Source: CAD feature listing. Evaluate the final solid. Frame: model axes, mm. Give positions to 0.01 mm unless a question says otherwise; leave off trailing zeros. Loops run counter-clockwise (first coordinate to the right, second up) from the corner with the lowest first, then second, coordinate; pieces in that order, holes last. Notation, with made-up numbers: M 37,32.5 L 66,32.5 A23 ccw 66,51.5 Z; hole C 52.5,-38 d4. An arc over 180 degrees is marked long. Put each result on its own line as item: value. Start each with the question number.
```python
from build123d import *

# Parameters (mm, degrees)
SKETCH_1_R          = 2
EXTRUDE_1_DEPTH     = 5
SKETCH_5_R          = 1.5
SKETCH_5_W          = 16.1
SKETCH_5_H          = 16.1
CUT_EXTRUDE_1_DEPTH = 4
EXTRUDE_2_DEPTH     = 5
FILLET_1_R          = 2
SKETCH_9_R          = 1.5
CUT_EXTRUDE_2_DEPTH = 10


with BuildPart() as part:
    # 草图1 → 凸台-拉伸1 (new body)
    with BuildSketch(Plane.XY):
        with BuildLine():
            Line((62.7093167, -58.345136948), (62.7093167, 57.654863052))
            ThreePointArc((62.7093167, 57.654863052), (62.123530262, 59.069076614), (60.7093167, 59.654863052))
            Line((60.7093167, 59.654863052), (-54.2906833, 59.654863052))
            ThreePointArc((-54.2906833, 59.654863052), (-55.704896862, 59.069076614), (-56.2906833, 57.654863052))
            Line((-56.2906833, 57.654863052), (-56.2906833, -58.345136948))
            ThreePointArc((-56.2906833, -58.345136948), (-55.704896862, -59.759350511), (-54.2906833, -60.345136948))
            Line((-54.2906833, -60.345136948), (60.7093167, -60.345136948))
            ThreePointArc((60.7093167, -60.345136948), (62.123530262, -59.759350511), (62.7093167, -58.345136948))
        make_face()
        with Locations((-52.2906833, -56.345136948)):
            Circle(SKETCH_1_R, mode=Mode.SUBTRACT)
        with Locations((58.7093167, -56.345136948)):
            Circle(SKETCH_1_R, mode=Mode.SUBTRACT)
        with Locations((58.7093167, 55.654863052)):
            Circle(SKETCH_1_R, mode=Mode.SUBTRACT)
        with Locations((-52.2906833, 55.654863052)):
            Circle(SKETCH_1_R, mode=Mode.SUBTRACT)
    extrude(amount=EXTRUDE_1_DEPTH)

    # 草图5 → 切除-拉伸1 (cut, through all)
    with BuildSketch(Plane.XY.offset(3)):
        with Locations((-48.275635297, 18.301860934)):
            Circle(SKETCH_5_R)
        with Locations((50.252991339, 18.301860934)):
            Circle(SKETCH_5_R)
        with Locations((-48.275635297, -6.698139066)):
            Circle(SKETCH_5_R)
        with Locations((50.252991339, -6.698139066)):
            Circle(SKETCH_5_R)
        with Locations((-48.275635297, -31.698139066)):
            Circle(SKETCH_5_R)
        with Locations((50.252991339, -31.698139066)):
            Circle(SKETCH_5_R)
        with Locations((25.214825615, -7.576393001)):
            Rectangle(SKETCH_5_W, SKETCH_5_H)
        with Locations((25.214825615, 14.423606999)):
            Rectangle(SKETCH_5_W, SKETCH_5_H)
        with Locations((3.214825615, -7.576393001)):
            Rectangle(SKETCH_5_W, SKETCH_5_H)
        with Locations((-18.785174385, 14.423606999)):
            Rectangle(SKETCH_5_W, SKETCH_5_H)
        with Locations((-18.785174385, -7.576393001)):
            Rectangle(SKETCH_5_W, SKETCH_5_H)
        with Locations((-18.785174385, -29.576393001)):
            Rectangle(SKETCH_5_W, SKETCH_5_H)
        with Locations((3.214825615, 14.423606999)):
            Rectangle(SKETCH_5_W, SKETCH_5_H)
        with Locations((3.214825615, -29.576393001)):
            Rectangle(SKETCH_5_W, SKETCH_5_H)
        with Locations((25.214825615, -29.576393001)):
            Rectangle(SKETCH_5_W, SKETCH_5_H)
        with Locations((25.214825615, -50.576393001)):
            Rectangle(SKETCH_5_W, SKETCH_5_H)
        with Locations((3.214825615, -50.576393001)):
            Rectangle(SKETCH_5_W, SKETCH_5_H)
        with Locations((-18.785174385, -50.576393001)):
            Rectangle(SKETCH_5_W, SKETCH_5_H)
    extrude(amount=-CUT_EXTRUDE_1_DEPTH, mode=Mode.SUBTRACT)

    # 草图8 → 凸台-拉伸2 (add)
    with BuildSketch(Plane.XY.offset(5)):
        Polygon((-56.2906833, -58.345136948), (-26.835174385, -58.345136948), (-26.835174385, -60.345136948), (33.264825615, -60.345136948), (33.264825615, -58.345136948), (62.7093167, -58.345136948), (62.7093167, -68.345136948), (33.264825615, -68.345136948), (-26.835174385, -68.345136948), (-56.2906833, -68.345136948), align=None)
    extrude(amount=-EXTRUDE_2_DEPTH)

    # 圆角1
    fillet_1_edges = [part.edges().sort_by_distance(p)[0] for p in [
        (-56.2906833, -68.345136948, 2.5),
        (62.7093167, -68.345136948, 2.5),
    ]]
    fillet(fillet_1_edges, radius=FILLET_1_R)

    # 草图9 → 切除-拉伸2 (cut)
    with BuildSketch(Plane(origin=(0, 0, 0), x_dir=(-1, 0, 0), z_dir=(0, 0, -1))):
        with Locations((-50.252991339, -6.698139066)):
            Circle(SKETCH_9_R)
        with Locations((-50.252991339, -31.698139066)):
            Circle(SKETCH_9_R)
        with Locations((48.275635297, -31.698139066)):
            Circle(SKETCH_9_R)
        with Locations((48.275635297, -6.698139066)):
            Circle(SKETCH_9_R)
        with Locations((48.275635297, 18.301860934)):
            Circle(SKETCH_9_R)
        with Locations((-50.252991339, 18.301860934)):
            Circle(SKETCH_9_R)
    extrude(amount=-CUT_EXTRUDE_2_DEPTH, mode=Mode.SUBTRACT)


solid = part.part
```
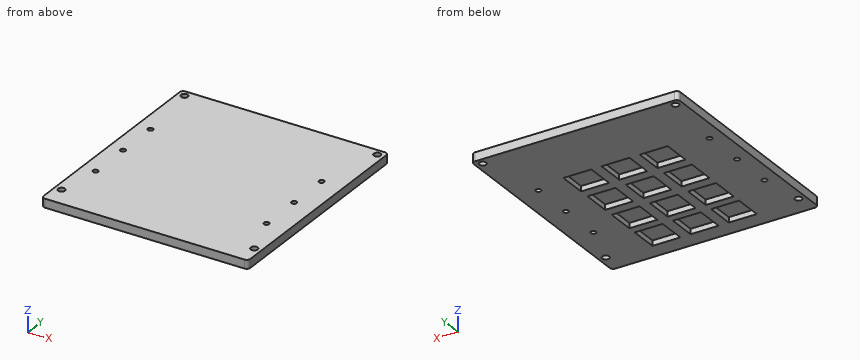
1. Section B-B, the plane y = -48. Output: boundary loops of the cut face in (x, z).
2. Contact query for flat-ended pins moving along their axis: pin 1 (1.8 mm diameter, centred on x = -48.28, y = -31.7, fed in from +Z); pin 2 (8 mm diameter, centred on x = 2, y = -8, fed in from -Z). Output: stop coordinate, or through.
3. Ray query, line 1 (Y direction, x = 4, z = 1.35); line 2 (X direction, y = -2.5, z = 2.55); line 3 (X direction, y = 18, z = 0.75). Return the intervals inside material, ascending.
4. Section C-C, the plane z = 1.45. State how many separate pieces and enclosed holes the cut face has, plus the area to 3 significant figures.
5. Section A-A, the plane x = 25.5. Output: boundary loops of the cut face in (y, z).
Results found:
1. outline: M -56.29,0 L -26.84,0 L -26.84,3 L -10.74,3 L -10.74,0 L -4.84,0 L -4.84,3 L 11.26,3 L 11.26,0 L 17.16,0 L 17.16,3 L 33.26,3 L 33.26,0 L 62.71,0 L 62.71,5 L -56.29,5 Z
2. pin 1: through
2. pin 2: z = 3
3. line 1: -68.35 to -58.63, -42.53 to -37.63, -21.53 to -15.63, 0.47 to 6.37, 22.47 to 59.65
3. line 2: -56.29 to -26.84, -10.74 to -4.84, 11.26 to 17.16, 33.26 to 62.71
3. line 3: -56.29 to -49.74, -46.81 to -26.84, -10.74 to -4.84, 11.26 to 17.16, 33.26 to 48.78, 51.72 to 62.71
4. separate pieces: 1
4. enclosed holes: 22
4. area: 12,000 mm²
5. outline: M -68.35,0 L -58.63,0 L -58.63,3 L -42.53,3 L -42.53,0 L -37.63,0 L -37.63,3 L -21.53,3 L -21.53,0 L -15.63,0 L -15.63,3 L 0.47,3 L 0.47,0 L 6.37,0 L 6.37,3 L 22.47,3 L 22.47,0 L 59.65,0 L 59.65,5 L -68.35,5 Z
